```python
from build123d import *

# Parameters (mm, degrees)
SKETCH_1_W             = 63
SKETCH_1_H             = 21.54
EXTRUDE_1_DEPTH        = 109.5
HOLE_WIZARD_M2_1_D     = 1.6
HOLE_WIZARD_M2_1_DEPTH = 5.2
HOLE_WIZARD_M2_1_TIP   = 0.480688495
SKETCH_4_R             = 2.5
EXTRUDE_2_DEPTH        = 4
SKETCH_5_R             = 7.414302321
SKETCH_5_R_2           = 4.881421022
CUT_EXTRUDE_1_DEPTH    = 2


with BuildPart() as part:
    # 草图1 → 凸台-拉伸1 (new body)
    with BuildSketch(Plane.XY):
        Rectangle(SKETCH_1_W, SKETCH_1_H)
    extrude(amount=EXTRUDE_1_DEPTH)

    # M2 螺纹孔1
    with Locations(Plane(origin=(0, -10.77, 0), x_dir=(-1, 0, 0), z_dir=(0, -1, 0))):
        with Locations((7, -105.2), (-7, -105.2), (-22.309756999, -30.762521908), (22.309756999, -30.762521908)):
            Hole(HOLE_WIZARD_M2_1_D / 2, depth=HOLE_WIZARD_M2_1_DEPTH)
            with Locations((0, 0, -(HOLE_WIZARD_M2_1_DEPTH + HOLE_WIZARD_M2_1_TIP / 2))):  # 118° drill point
                Cone(0, HOLE_WIZARD_M2_1_D / 2, HOLE_WIZARD_M2_1_TIP, mode=Mode.SUBTRACT)

    # 草图4 → 凸台-拉伸2 (add)
    with BuildSketch(Plane.XY.offset(109.5)):
        with Locations((-6, -6.77)):
            Circle(SKETCH_4_R)
        with Locations((6, -6.77)):
            Circle(SKETCH_4_R)
    extrude(amount=EXTRUDE_2_DEPTH)

    # 草图5 → 切除-拉伸1 (cut)
    with BuildSketch(Plane(origin=(0, 0, 0), x_dir=(-1, 0, 0), z_dir=(0, 0, -1))):
        Circle(SKETCH_5_R)
        Circle(SKETCH_5_R_2, mode=Mode.SUBTRACT)
    extrude(amount=-CUT_EXTRUDE_1_DEPTH, mode=Mode.SUBTRACT)


solid = part.part
```
Verification items for the finished model (mm, model axes). A direction names the side the tool comes from. Coordinates: 2 decimals unless noted, no trailing zeros. Write each loop counter-clockwise with the first axis right and the second up, starting at its lowest first coordinate (ties: lowest second). Pieces come first, ordered by that corner, then holes. Notation, with made-up numbers: (75.5, 58.25) - (111.5, 58.25) arc R14 cw to (111.5, 69.25) - close; hole circle Ø8 at (87.5, -24). An arc over 180 degrees is marked (long way). Write item = value, one per line.
Q1. Mould release check, pull along Y, two halves, no side actions. Record for faces 4 (the face through (0, 10.77, 54)), 5 (the face through (-2, -5, 2)), 6 (the face through (0, 0, 109.5)), 7 (the face through (5.465, 5.011, 0.986)): released by +Y, released by -Y, zero draft, split by the parting line, or undercut.
Answer:
face_4 = released by +Y
face_5 = undercut
face_6 = zero draft
face_7 = undercut
Q2. Material ranges on L1, parallel to X at y = -7.8, z = 105.2; L2, parallel to Y at x = 0, z = 1.35; L3, parallel to Z at x = -7, y = -8.1, recorded low to high. Write a range as from..to.
Answer:
L1 = -31.5..-7.8, -6.2..6.2, 7.8..31.5
L2 = -10.77..-7.41, -4.88..4.88, 7.41..10.77
L3 = 0..104.4, 106..113.5
Q3. Cross-section at A-A (x = 0). Enter the section's corners in (y, z), plus the area to 3 significant figures.
Answer:
outline = (-10.77, 0) - (-7.41, 0) - (-7.41, 2) - (-4.88, 2) - (-4.88, 0) - (4.88, 0) - (4.88, 2) - (7.41, 2) - (7.41, 0) - (10.77, 0) - (10.77, 109.5) - (-10.77, 109.5) - close
area = 2,350 mm²
Q4. Go/stop test with flat-tipped pins: pin 1 Ø3 at (x, y) = (11.5, -2.5) entering from +Z; pin 2 Ø10 at (x, y) = (4, -1.5) entering from +Z; pin 3 Ø1.4 at (x, z) = (-7, 105.2) entering from -Y. Record where each tip stops, or that it passes through.
Answer:
pin_1 = 109.5
pin_2 = 113.5
pin_3 = -5.51
Q5. Access from +Z, -Z, +X, -X, +Y, -Y to the whole of each face (thin tool, end or side, straight path). Record for faces 1 (the face through (3.874, -2.97, 0.986)), 2 (the face through (0, 0, 0)), 3 (the face through (-3.615, -6.019, 111.472)).
Answer:
face_1 = -Z
face_2 = -Z, +X, -X, +Y, -Y
face_3 = +Z
Q6. Cross-section at B-B (y = 0). Enter the section's corners in (x, z).
Answer:
outline = (-31.5, 0) - (-7.41, 0) - (-7.41, 2) - (-4.88, 2) - (-4.88, 0) - (4.88, 0) - (4.88, 2) - (7.41, 2) - (7.41, 0) - (31.5, 0) - (31.5, 109.5) - (-31.5, 109.5) - close
Q7. Cross-section at C-C (x = 12.5). Enter the section's corners in (y, z).
Answer:
outline = (-10.77, 0) - (10.77, 0) - (10.77, 109.5) - (-10.77, 109.5) - close
